from build123d import *

# Parameters (mm, degrees)
SKETCH1_R           = 15
SKETCH1_R_2         = 7.5
BOSS_EXTRUDE1_DEPTH = 20
FILLET1_R           = 10
BOSS_EXTRUDE3_START = 10
SKETCH2_R           = 10
BOSS_EXTRUDE3_DEPTH = 80
SKETCH5_R           = 7.5
CUT_EXTRUDE3_DEPTH  = 30


with BuildPart() as part:
    # Sketch1 → Boss-Extrude1 (new body)
    with BuildSketch(Plane.XY):
        Circle(SKETCH1_R)
        Circle(SKETCH1_R_2, mode=Mode.SUBTRACT)
    extrude(amount=BOSS_EXTRUDE1_DEPTH)

    # Fillet1
    # the kernel refuses this fillet: 10 mm, written as the material it takes off along each edge
    with BuildSketch(Plane(origin=(0, 0, 0), x_dir=(1, 0, 0), z_dir=(0, -1, 0))) as fillet1_piece_1:
        with BuildLine():
            CenterArc((5, 9.682458366), FILLET1_R, 284.477512186, 75.522487814)
            Line((7.5, 0), (7.55, -0.193649167))
            ThreePointArc((7.55, -0.193649167), (11.25, -0.2), (15, -0.2))
            Line((15, -0.2), (15.2, 0))
            Line((15.2, 0), (15.2, 9.682458366))
            Line((15.2, 9.682458366), (15, 9.682458366))
        make_face()
    revolve(axis=Axis((0, 0, 0), (0, 0, 1)), mode=Mode.SUBTRACT)
    with BuildSketch(Plane(origin=(0, 0, 20), x_dir=(1, 0, 0), z_dir=(0, -1, 0))) as fillet1_piece_2:
        with BuildLine():
            CenterArc((5, -9.682458366), FILLET1_R, 0, 75.522487814)
            Line((7.5, 0), (7.55, 0.193649167))
            ThreePointArc((7.55, 0.193649167), (11.25, 0.2), (15, 0.2))
            Line((15, 0.2), (15.2, 0))
            Line((15.2, 0), (15.2, -9.682458366))
            Line((15.2, -9.682458366), (15, -9.682458366))
        make_face()
    revolve(axis=Axis((0, 0, 20), (0, 0, 1)), mode=Mode.SUBTRACT)

    # Sketch2 → Boss-Extrude3 (add)
    with BuildSketch(Plane(origin=(0, 0, 0), x_dir=(1, 0, 0), z_dir=(0, 1, 0)).offset(BOSS_EXTRUDE3_START)):
        with Locations(Location((0, -10, 0), (0, 0, 47.908263914))):
            Circle(SKETCH2_R)
    extrude(amount=BOSS_EXTRUDE3_DEPTH)

    # Sketch5 → Cut-Extrude3 (cut)
    with BuildSketch(Plane(origin=(0, 90, 0), x_dir=(1, 0, 0), z_dir=(0, 1, 0))):
        with Locations(Location((0, -10, 0), (0, 0, 270))):
            Circle(SKETCH5_R)
    extrude(amount=-CUT_EXTRUDE3_DEPTH, mode=Mode.SUBTRACT)


solid = part.part
Source: CAD feature listing. Evaluate the final solid. Frame: model axes, mm. A direction names the side the tool comes from. Coordinates: 2 decimals unless noted, no trailing zeros. Write each loop counter-clockwise with the first axis right and the second up, starting at its lowest first coordinate (ties: lowest second). Pieces come first, ordered by that corner, then holes. Notation, with made-up numbers: M 68,-26 L 72,-26 A33 cw 72,9 Z; hole C -40,40 d8. An arc over 180 degrees is marked long. Use a Markdown table: item, result.
1) Section A-A, the plane y = 42. Output: boundary loops of the cut face in (x, z).
Conclusion:
| item | result |
|---|---|
| outline | C 0,10 d20 |
2) Ray query, L1, parallel to Y at x = 0, z = 9.5; L2, parallel to X at y = 68.5, z = 10; L3, parallel to Z at x = -5, y = 69.5. Return the intervals inside material, ascending.
Conclusion:
| item | result |
|---|---|
| L1 | y = -15 to -7.5, 7.5 to 60 |
| L2 | x = -10 to -7.5, 7.5 to 10 |
| L3 | z = 1.34 to 4.41, 15.59 to 18.66 |
3) Reachability of faces 4 (the cylindrical face through (0.33, 75.21, 2.507)), 5 (the cylindrical face through (-0.51, -14.99, 10)) from +Z, -Z, +X, -X, +Y, -Y: full face, straight path, thin tool, end or side. Return the list, or none.
Conclusion:
| item | result |
|---|---|
| face 4 | +Y |
| face 5 | +Z, -Z |
4) Mould query, pull axis Z, two halves, no side actions, for faces 1 (the cylindrical face through (-0.804, 49.44, 19.968)), 2 (the flat face through (0, 60, 10)), 3 (the cylindrical face through (-7.493, 0.33, 9.86)). Classes: pulls with the +Z half, pulls with the -Z half, needs draft (parallel to the pull), parting line crosses it, or undercut.
Conclusion:
| item | result |
|---|---|
| face 1 | parting line crosses it |
| face 2 | undercut |
| face 3 | needs draft |
5) First-contact query: pin 1 Ø1.5 at (y, z) = (6, 8) entering from -X; pin 2 Ø1.3 at (x, z) = (1.5, 18.5) entering from -Y; pin 3 Ø6 at (x, y) = (-11.5, 46) entering from -Z; pin 4 Ø13.5 at (x, y) = (0, 0) entering from +Z. Flat tips, straight axial feed; report the tip coordinate or a pass-through.
Conclusion:
| item | result |
|---|---|
| pin 1 | stops at x = -13.93 |
| pin 2 | stops at y = -11.48 |
| pin 3 | stops at z = 4.73 |
| pin 4 | passes through |
